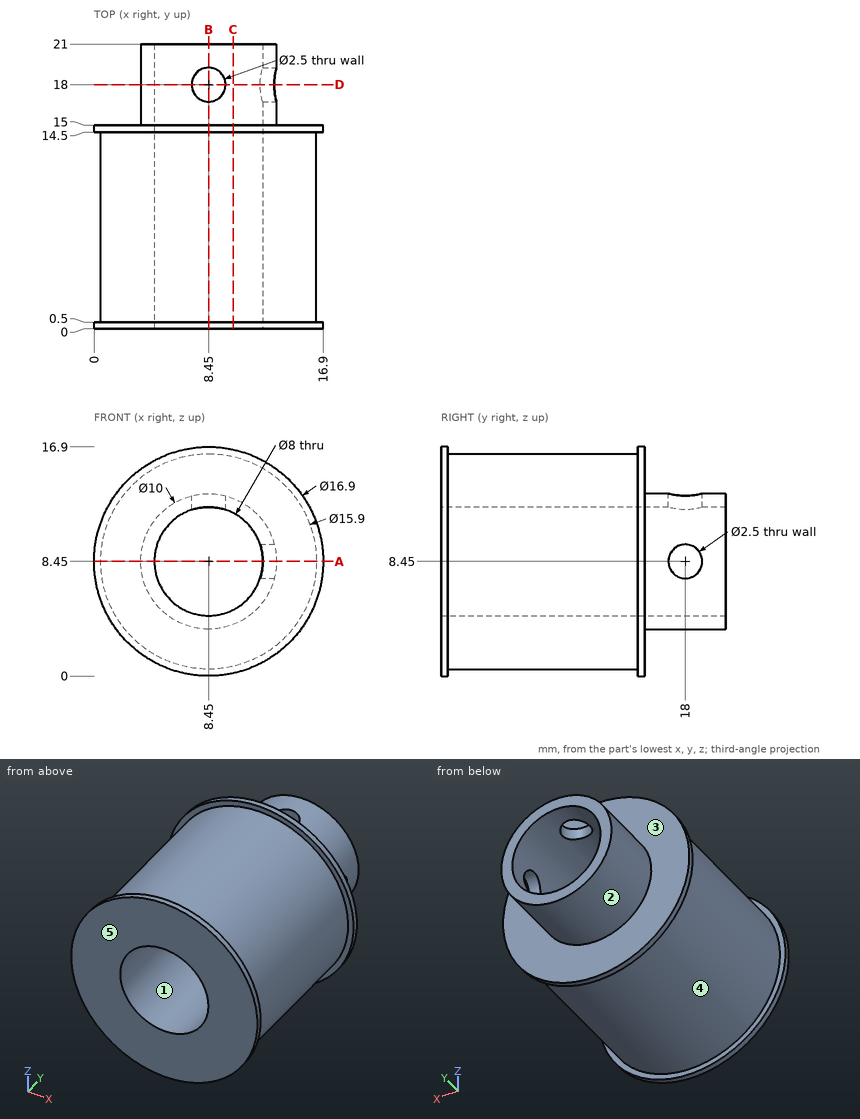
Check sheet for the drawn part. Datum: minimum x, y, z corner. Units: mm. A direction names the side the tool comes from. Round coordinates to 2 decimals unless told otherwise and drop trailing zeros. Write each loop counter-clockwise with the first axis right and the second up, starting at its lowest first coordinate (ties: lowest second). Pieces come first, ordered by that corner, then holes. Notation, with made-up numbers: (-33.5, 75.25) -> (-23.5, 75.25) arc R22 cw to (-23.5, 90.25) -> close; hole circle Ø10 at (78.5, 73). An arc over 180 degrees is marked (long way). Put each result on its own line as item: value.
(1) Tool access check on the marked faces 1 and 2. Record the directions out of +Z, -Z, +X, -X, +Y, -Y that give a thin tool (end or side, any length) a straight path to the whole face; none if there is none.
Values found:
face 1: +Y, -Y
face 2: +Y
(2) Mould release check, pull along Y, two halves, no side actions. Record for the marked faces 3, 4 and 5: released by +Y, released by -Y, zero draft, split by the parting line, or undercut.
Values found:
face 3: released by +Y
face 4: undercut
face 5: released by -Y
(3) Material ranges on line 1 (Y direction, x = 12.7, z = 8.45); line 2 (X direction, y = 16.5, z = 8.45); line 3 (X direction, y = 13.25, z = 8.45), recorded low to high.
Values found:
line 1: y = 0 to 16.75, 19.25 to 21
line 2: x = 3.45 to 4.45, 12.45 to 13.45
line 3: x = 0.5 to 4.45, 12.45 to 16.4
(4) Sectioned sample at D-D (y = 18). Enter the section's corners in (x, z), plus the area to 3 significant figures.
Values found:
outline: (7.2, 12.25) -> (7.2, 13.29) arc R5 ccw (long way) to (13.29, 7.2) -> (12.25, 7.2) arc R4 cw (long way) to start; (9.7, 12.25) arc R4 cw to (12.25, 9.7) -> (13.29, 9.7) arc R5 ccw to (9.7, 13.29) -> close
area: 23.2 mm^2
(5) Sectioned sample at A-A (z = 8.45). Enter the section's corners in (x, y).
Values found:
outline: (0, 0) -> (4.45, 0) -> (4.45, 21) -> (3.45, 21) -> (3.45, 15) -> (0, 15) -> (0, 14.5) -> (0.5, 14.5) -> (0.5, 0.5) -> (0, 0.5) -> close; (12.45, 0) -> (16.9, 0) -> (16.9, 0.5) -> (16.4, 0.5) -> (16.4, 14.5) -> (16.9, 14.5) -> (16.9, 15) -> (13.45, 15) -> (13.45, 16.75) -> (12.45, 16.75) -> close; (12.45, 19.25) -> (13.45, 19.25) -> (13.45, 21) -> (12.45, 21) -> close
(6) Sectioned sample at B-B (x = 8.45). Enter the section's corners in (y, z).
Values found:
outline: (0, 0) -> (0.5, 0) -> (0.5, 0.5) -> (14.5, 0.5) -> (14.5, 0) -> (15, 0) -> (15, 3.45) -> (21, 3.45) -> (21, 4.45) -> (0, 4.45) -> close; (0, 12.45) -> (16.75, 12.45) -> (16.75, 13.45) -> (15, 13.45) -> (15, 16.9) -> (14.5, 16.9) -> (14.5, 16.4) -> (0.5, 16.4) -> (0.5, 16.9) -> (0, 16.9) -> close; (19.25, 12.45) -> (21, 12.45) -> (21, 13.45) -> (19.25, 13.45) -> close
(7) Sectioned sample at C-C (x = 10.25). Enter the section's corners in (y, z), plus the area to 3 significant figures.
Values found:
outline: (0, 0.19) -> (0.5, 0.19) -> (0.5, 0.71) -> (14.5, 0.71) -> (14.5, 0.19) -> (15, 0.19) -> (15, 3.79) -> (21, 3.79) -> (21, 4.88) -> (0, 4.88) -> close; (0, 12.02) -> (21, 12.02) -> (21, 13.11) -> (15, 13.11) -> (15, 16.71) -> (14.5, 16.71) -> (14.5, 16.19) -> (0.5, 16.19) -> (0.5, 16.71) -> (0, 16.71) -> close
area: 139 mm^2
(8) Go/stop test with flat-tipped pins: pin 1 Ø2 at (y, z) = (4.5, 2) entering from -X; pin 2 Ø10 at (x, y) = (2, 12.5) entering from +Z; pin 3 Ø3 at (x, y) = (14.5, 9.5) entering from -Z; pin 4 Ø6.5 at (x, z) = (8.45, 8.45) entering from +Y. Record where each tip stops, or that it passes through.
Values found:
pin 1: stops at x = 2.66
pin 2: stops at z = 16.69
pin 3: stops at z = 1.93
pin 4: passes through
